Here's how the part is built. I have some questions about the finished solid (model axes, mm). Face numbers are marked on the shaded views. A direction names the side the tool comes from. Round coordinates to 2 decimals unless told otherwise and drop trailing zeros. Write each loop counter-clockwise with the first axis right and the second up, starting at its lowest first coordinate (ties: lowest second). Pieces come first, ordered by that corner, then holes. Notation, with made-up numbers: (-13.5, -29) - (32.5, -29) arc R32 cw to (32.5, -2) - close; hole circle Ø11 at (-37, 55.25). An arc over 180 degrees is marked (long way). One line per item, written item: value. Start each with the question number.
Item 1: Imagine slicing it at D-D, the plane x = -2.5. Please give me the cut outline in (y, z), then the cut area to 3 significant figures.
Item 2: Imagine slicing it at A-A, the plane y = -22. Please give me the cut outline in (x, z).
Item 3: Imagine slicing it at B-B, the plane z = 17. Please give me the cut outline in (x, y), then the cut area to 3 significant figures.
Item 4: For P1, Ø3, axis at y = -7.5, z = 19.5, coming from the -X side; P2, Ø5, axis at y = -35.5, z = 17, coming from the +X side; P3, Ø8, axis at x = 9.5, y = -13, coming from the -Z side, each with a flat end and sliding along its axis, tell me the tip position at first contact or that it passes through.
Item 5: Thinking about a two-plate mould opening in Y: for the marked faces 1, 2 and 3, which applies, released by +Y, released by -Y, zero draft, split by the parting line, or undercut?
Item 6: If I drill on line 1 (Y direction, x = 11.5, z = 0.5); line 2 (Z direction, x = 3, y = 13); line 3 (X direction, y = -16.5, z = -8), over which ranges is the centre line in solid material (lowest first)?
Item 7: Imagine slicing it at C-C, the plane x = 9. Please give me the cut outline in (y, z), then the cut area to 3 significant figures.
Item 8: For the marked faces 4, 5 and 6, which set-ups out of +Z, -Z, +X, -X, +Y, -Y let a thin tool reach every point of the face, with its end or its side?
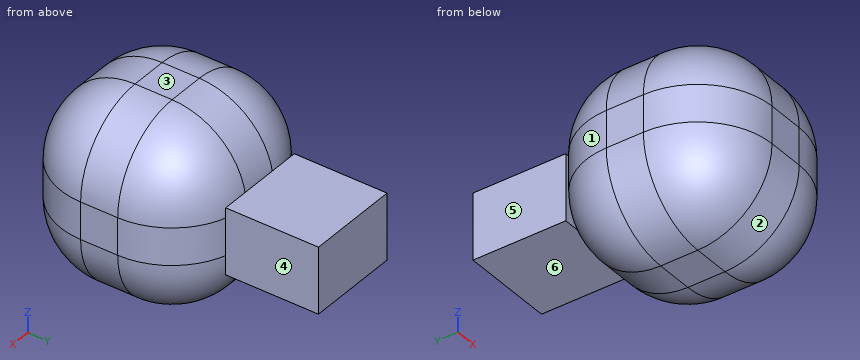
```python
from build123d import *

# Parameters (mm, degrees)
F0_W     = 50
F0_H     = 50
F1_DEPTH = 50
F2_R     = 20
F3_W     = 25.187926
F3_H     = 17.857752
F4_DEPTH = 25


with BuildPart() as f1:
    # F0 (on Front) → F1 (new body)
    with BuildSketch(Plane.XZ):
        Rectangle(F0_W, F0_H)
    extrude(amount=F1_DEPTH)

    # F2
    f2_edges = [f1.edges().sort_by_distance(p)[0] for p in [
        (25, 0, 0),
        (-25, 0, 0),
        (25, -50, 0),
        (25, -25, 25),
        (-25, -25, 25),
        (0, 0, 25),
        (0, -50, 25),
        (-25, -50, 0),
        (0, -50, -25),
        (-25, -25, -25),
        (0, 0, -25),
        (25, -25, -25),
    ]]
    fillet(f2_edges, radius=F2_R)

    # F3 (on Front) → F4 (join)
    with BuildSketch(Plane.XZ):
        Rectangle(F3_W, F3_H)
    extrude(amount=-F4_DEPTH)


solid = f1.part
```
Values follow:
1. outline: (-50, -5) arc R20 ccw to (-30, -25) - (-20, -25) arc R20 ccw to (0, -5) - (0, -8.93) - (25, -8.93) - (25, 8.93) - (0, 8.93) - (0, 5) arc R20 ccw to (-20, 25) - (-30, 25) arc R20 ccw to (-50, 5) - close
1. area: 2,600 mm^2
2. outline: (-25, -5) arc R20 ccw to (-5, -25) - (5, -25) arc R20 ccw to (25, -5) - (25, 5) arc R20 ccw to (5, 25) - (-5, 25) arc R20 ccw to (-25, 5) - close
3. outline: (-21, -30) arc R16 ccw to (-5, -46) - (5, -46) arc R16 ccw to (21, -30) - (21, -20) arc R16 ccw to (5, -4) - (-5, -4) arc R16 ccw to (-21, -20) - close
3. area: 1,540 mm^2
4. P1: stops at x = -14.42
4. P2: stops at x = 21.9
4. P3: stops at z = -24.53
5. face 1: undercut
5. face 2: released by -Y
5. face 3: zero draft
6. line 1: y = -48.91 to -1.09, 0 to 25
6. line 2: z = -8.93 to 8.93
6. line 3: x = -24.46 to 24.46
7. outline: (-49.6, -5) arc R19.6 ccw to (-30, -24.6) - (-20, -24.6) arc R19.6 ccw to (-0.4, -5) - (-0.4, 5) arc R19.6 ccw to (-20, 24.6) - (-30, 24.6) arc R19.6 ccw to (-49.6, 5) - close; (0, -8.93) - (25, -8.93) - (25, 8.93) - (0, 8.93) - close
7. area: 2,540 mm^2
8. face 4: +Z, -Z, +X, +Y
8. face 5: +Z, -Z, -X, +Y
8. face 6: -Z, +X, -X, +Y
